Read the model definition and answer for the solid it produces. Units are mm, in the model's axes. Round coordinates to 2 decimals unless told otherwise and drop trailing zeros. Order: outer loops, then holes, each group sorted by start corner. A loop starts at its lowest first (then second) coordinate and runs counter-clockwise, first axis right, second up.
from build123d import *

# Parameters (mm, degrees)
SKETCH3_W           = 180
SKETCH3_H           = 180
SKETCH3_W_2         = 3.18
SKETCH3_H_2         = 20
BOSS_EXTRUDE1_DEPTH = 3.18
CUT_EXTRUDE1_DEPTH  = 128.318939675
SKETCH5_R           = 1.436023081
SKETCH5_W           = 3.18
SKETCH5_H           = 80.125
CUT_EXTRUDE2_DEPTH  = 128.318939675


with BuildPart() as part:
    # Sketch3 → Boss-Extrude1 (new body)
    with BuildSketch(Plane.XY):
        Rectangle(SKETCH3_W, SKETCH3_H)
        with Locations((46.269729843, -0.125)):
            Rectangle(SKETCH3_W_2, SKETCH3_H_2, mode=Mode.SUBTRACT)
    extrude(amount=BOSS_EXTRUDE1_DEPTH)

    # Sketch4 → Cut-Extrude1 (cut, through all)
    with BuildSketch(Plane.XY.offset(3.18)):
        Polygon((1.5, 86.82), (10, 86.82), (10, 90), (-10, 90), (-10, 86.82), (-1.5, 86.82), (-1.5, 82.82), (-3.5, 82.82), (-3.5, 79.82), (-1.5, 79.82), (-1.5, 77), (1.5, 77), (1.5, 79.82), (3.5, 79.82), (3.5, 82.82), (1.5, 82.82), align=None)
        Polygon((1.5, -79.82), (1.5, -77), (-1.5, -77), (-1.5, -79.82), (-3.5, -79.82), (-3.5, -82.82), (-1.5, -82.82), (-1.5, -86.82), (-10, -86.82), (-10, -90), (10, -90), (10, -86.82), (1.5, -86.82), (1.5, -82.82), (3.5, -82.82), (3.5, -79.82), align=None)
    extrude(amount=-CUT_EXTRUDE1_DEPTH, mode=Mode.SUBTRACT)

    # Sketch5 → Cut-Extrude2 (cut, through all)
    with BuildSketch(Plane.XY.offset(3.18)):
        with Locations((-88, 0)):
            Circle(SKETCH5_R)
        with Locations((88, 0)):
            Circle(SKETCH5_R)
        with Locations((-88.41, 49.9375)):
            Rectangle(SKETCH5_W, SKETCH5_H)
        with Locations((-88.41, -49.9375)):
            Rectangle(SKETCH5_W, SKETCH5_H)
        with Locations((88.41, -49.9375)):
            Rectangle(SKETCH5_W, SKETCH5_H)
        with Locations((88.41, 49.9375)):
            Rectangle(SKETCH5_W, SKETCH5_H)
    extrude(amount=-CUT_EXTRUDE2_DEPTH, mode=Mode.SUBTRACT)


solid = part.part
Q1. A cutting plane is placed at B-B, the plane z = 2.45. Give the number of separate pieces and of enclosed holes in the cut face, plus the area to 3 significant figures.
Outcome:
separate pieces: 1
enclosed holes: 3
area: 31,100 mm2
Q2. Flat-ended cylindrical pins translate along their axes: pin 1 (1 mm diameter, centred on x = 5.5, z = 1.5, fed in from -Y); pin 2 (1.6 mm diameter, centred on x = -89, z = 1.5, fed in from -Y) (3 decimals); pin 3 (1.6 mm diameter, centred on y = -88, z = 2, fed in from -X). Find the tip coordinate at first contact, or state that the pin passes through.
Outcome:
pin 1: stops at y = -86.82
pin 2: stops at y = -9.875
pin 3: stops at x = -86.82
Q3. Straight lines are drawn through the part: probe 1 along Y at (x, z) = (-88, 1.85) (3 decimals); probe 2 along X at (y, z) = (5, 1.4); probe 3 along Y at (x, z) = (-6.5, 1.65). For each, find the intervals that lie inside material, in ascending order.
Outcome:
probe 1: y = -9.875 to -1.436, 1.436 to 9.875
probe 2: x = -90 to 44.68, 47.86 to 90
probe 3: y = -86.82 to 86.82
Q4. A cutting plane is placed at A-A, the plane y = -33.5. Give the vertices of the cut face in (x, z), plus the area to 3 significant figures.
Outcome:
outline: (-86.82, 0) - (86.82, 0) - (86.82, 3.18) - (-86.82, 3.18) - close
area: 552 mm2
